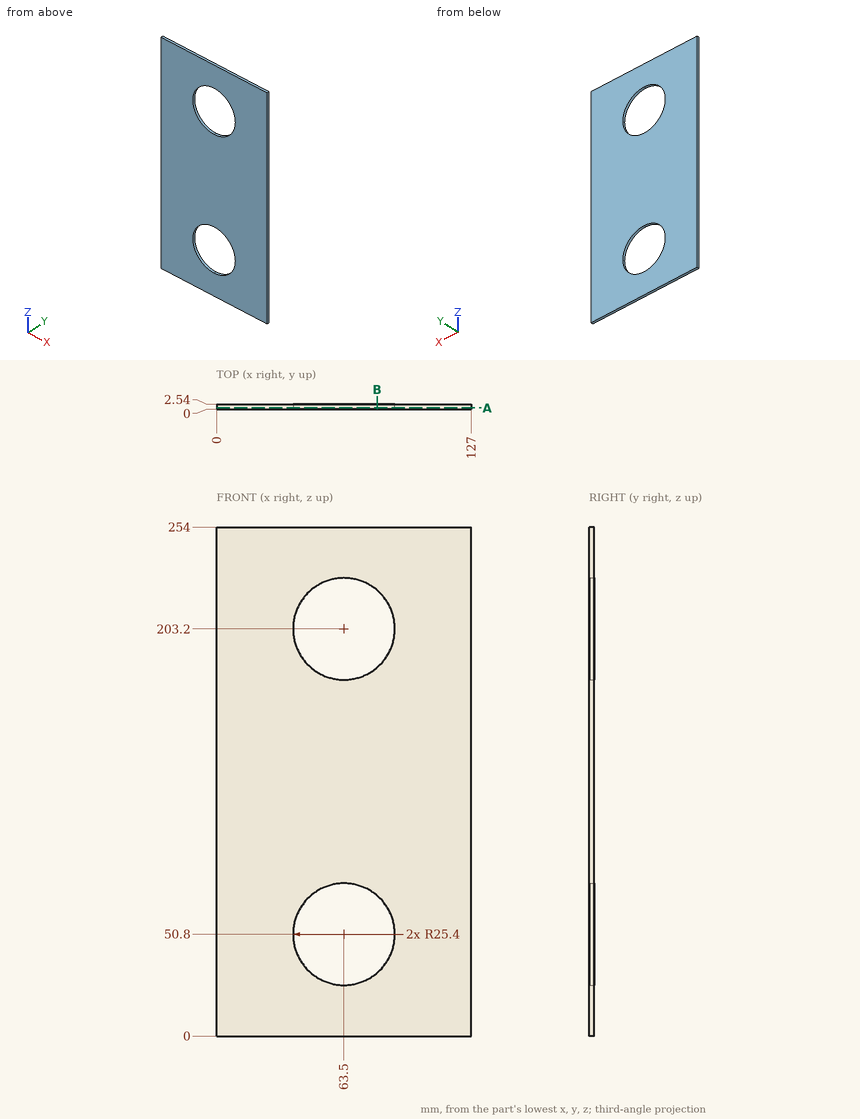
Part print with two shaded views. Sizes in mm from the minimum x, y, z corner. Give positions to 0.01 mm unless a question says otherwise; leave off trailing zeros. Order: outer loops, then holes, each group sorted by start corner. A loop starts at its lowest first (then second) coordinate and runs counter-clockwise, first axis right, second up. Notation, with made-up numbers: M 40,-14.75 L 79,-14.75 A18 cw 79,19.25 Z; hole C -9.75,-11 d5. An arc over 180 degrees is marked long. Write item = value, one per line.
Q1. Cut at A-A, the plane y = 0.65. List the corners of the cut face in (x, z).
Derived:
outline = M 0,0 L 127,0 L 127,254 L 0,254 Z; hole M 63.5,25.4 A25.4 ccw 88.9,50.8 A25.4 ccw long Z; hole M 63.5,177.8 A25.4 ccw 88.9,203.2 A25.4 ccw long Z
Q2. Flat gauge pin, fed straight in: pin 1 (1 mm diameter, centred on x = 103, y = 1.5, fed in from -Z). Where does the tip first touch, or does it go through?
Derived:
pin_1 = 0
Q3. Drill centre lines: line 1 (Z direction, x = 62.5, y = 0.7); line 2 (Z direction, x = 57.5, y = 1.55); line 3 (X direction, y = 2.4, z = 38.5). Where is each one in solid material? Low to high. Write a range as [from, to].
Derived:
line_1 = [0, 25.42], [76.18, 177.82], [228.58, 254]
line_2 = [0, 26.12], [75.48, 178.52], [227.88, 254]
line_3 = [0, 41.28], [85.72, 127]
Q4. Cut at B-B, the plane x = 80. List the corners of the cut face in (y, z).
Derived:
outline = M 0,0 L 2.54,0 L 2.54,31.49 L 0,31.49 Z; M 0,70.11 L 2.54,70.11 L 2.54,183.89 L 0,183.89 Z; M 0,222.51 L 2.54,222.51 L 2.54,254 L 0,254 Z
